Verification items for the finished model (mm, model axes). A direction names the side the tool comes from. Give positions to 0.01 mm unless a question says otherwise; leave off trailing zeros. Loops run counter-clockwise (first coordinate to the right, second up) from the corner with the lowest first, then second, coordinate; pieces in that order, holes last. Notation, with made-up numbers: (61, 56) - (97, 56) arc R12 ccw to (97, 79) - close; hole circle Ø2 at (-9, -10.5). An arc over 180 degrees is marked (long way). One line per item, written item: value. Start each with the question number.
1. Access from +Z, -Z, +X, -X, +Y, -Y to the whole of each face (thin tool, end or side, straight path). Record for faces 4 (the flat face through (-7.445, -14, -16)), 5 (the flat face through (-19, 0, -10)), 6 (the flat face through (-19, 0, 0)).
2. Sectioned sample at B-B (y = 5). Record the cut outline in (x, z).
3. Mould release check, pull along X, two halves, no side actions. Record for faces 1 (the cylindrical face through (-36.438, 27.629, -4.93)), 2 (the flat face through (-2.4, -9.8, -20.5)), 3 (the cylindrical face through (-26.078, 9.817, -4.93)): pulls with the +X half, pulls with the -X half, needs draft (parallel to the pull), parting line crosses it, or undercut.
4. Sectioned sample at C-C (z = -8.5). Record the cut outline in (x, y), plus the area to 3 significant figures.
5. Gauge pin test, flat ends, axial feed: pin 1 (12 mm diameter, centred on x = -25.5, y = -11, fed in from -Z); pin 2 (5 mm diameter, centred on y = -11, z = -20, fed in from -X); pin 3 (3 mm diameter, centred on x = -34.5, z = -4.5, fed in from +Y); pin 4 (12 mm diameter, centred on x = -18.44, y = 9.48, fed in from -Z). Record the tip position at first contact, or that the pin passes through.
6. Sectioned sample at D-D (x = -13.5). Record the cut outline in (y, z).
7. Sectioned sample at A-A (x = -19). Record the cut outline in (y, z), plus the area to 3 significant figures.
8. Scan lines: L1, parallel to Z at x = -24, y = 28.5; L2, parallel to X at y = -3, z = -11; L3, parallel to X at y = 15, z = -2.5. Record each from-to range of solid material in increasing order. Write a range as [from, to].
from build123d import *

# Parameters (mm, degrees)
SKETCH1_R           = 7.64
SKETCH1_R_2         = 4.14
BOSS_EXTRUDE1_DEPTH = 10
BOSS_EXTRUDE2_DEPTH = 10


with BuildPart() as part:
    # Sketch1 → Boss-Extrude1 (new body)
    with BuildSketch(Plane.XY):
        with BuildLine():
            Line((-7.444896481, 30.480652594), (-29.444896481, 30.480652594))
            ThreePointArc((-29.444896481, 30.480652594), (-36.515964293, 27.551720406), (-39.444896481, 20.480652594))
            Line((-39.444896481, 20.480652594), (-39.444896481, -20.519347406))
            Line((-39.444896481, -20.519347406), (2.555103519, -20.519347406))
            Line((2.555103519, -20.519347406), (2.555103519, 20.480652594))
            ThreePointArc((2.555103519, 20.480652594), (-0.373828669, 27.551720406), (-7.444896481, 30.480652594))
        make_face()
        with Locations((-18.444896481, 9.480652594)):
            Circle(SKETCH1_R, mode=Mode.SUBTRACT)
        with Locations((-18.444896481, -11.019347406)):
            Circle(SKETCH1_R_2, mode=Mode.SUBTRACT)
    extrude(amount=-BOSS_EXTRUDE1_DEPTH)

    # Sketch2 → Boss-Extrude2 (add)
    with BuildSketch(Plane(origin=(2.555103519, 0, 0), x_dir=(0, 0, -1), z_dir=(1, 0, 0))):
        Polygon((10, 0.69821188), (31.217559285, -20.519347406), (10, -20.519347406), align=None)
    extrude(amount=-BOSS_EXTRUDE2_DEPTH)


solid = part.part
Results are:
1. face 4: -Z, -X, +Y, -Y
1. face 5: -Z, -X, +Y
1. face 6: +Z, +X, -X, +Y, -Y
2. outline: (-39.44, -10) - (-24.63, -10) - (-24.63, 0) - (-39.44, 0) - close; (-12.26, -10) - (2.56, -10) - (2.56, 0) - (-12.26, 0) - close
3. face 1: pulls with the -X half
3. face 2: needs draft
3. face 3: undercut
4. outline: (-39.44, -20.52) - (2.56, -20.52) - (2.56, 20.48) arc R10 ccw to (-7.44, 30.48) - (-29.44, 30.48) arc R10 ccw to (-39.44, 20.48) - close; hole circle Ø15.28 at (-18.44, 9.48); hole circle Ø8.28 at (-18.44, -11.02)
4. area: 1,860 mm^2
5. pin 1: stops at z = -10
5. pin 2: stops at x = -7.44
5. pin 3: stops at y = 29.83
5. pin 4: passes through
6. outline: (-20.52, -10) - (3.66, -10) - (3.66, 0) - (-20.52, 0) - close; (15.3, -10) - (30.48, -10) - (30.48, 0) - (15.3, 0) - close
7. outline: (-20.52, -10) - (-15.12, -10) - (-15.12, 0) - (-20.52, 0) - close; (-6.92, -10) - (1.86, -10) - (1.86, 0) - (-6.92, 0) - close; (17.1, -10) - (30.48, -10) - (30.48, 0) - (17.1, 0) - close
7. area: 276 mm^2
8. L1: z = [-10, 0]
8. L2: x = [-7.44, 2.56]
8. L3: x = [-39.44, -23.73], [-13.16, 2.56]
